```python
from build123d import *

# Parameters (mm, degrees)
F0_R     = 44
F1_DEPTH = 2
F0_R_2   = 1.5
F2_DEPTH = 1


# Not quite as in the source:
# - a fillet or chamfer that OpenCascade refuses, or shapes differently, is made with other operations: its cross-section is extruded or revolved along the edge and cut away or added


with BuildPart() as f1:
    # F0 (on Front) → F1 (new body)
    with BuildSketch(Plane.XZ):
        with BuildLine():
            Line((-77.5, -50), (77.5, -50))
            Line((77.5, -50), (77.5, -40))
            Line((77.5, -40), (72.5, -40))
            ThreePointArc((72.5, -40), (67.5, -35), (72.5, -30))
            Line((72.5, -30), (77.5, -30))
            Line((77.5, -30), (77.5, 30))
            Line((77.5, 30), (72.5, 30))
            ThreePointArc((72.5, 30), (67.5, 35), (72.5, 40))
            Line((72.5, 40), (77.5, 40))
            Line((77.5, 40), (77.5, 50))
            Line((77.5, 50), (-77.5, 50))
            Line((-77.5, 50), (-77.5, 40))
            Line((-77.5, 40), (-72.5, 40))
            ThreePointArc((-72.5, 40), (-67.5, 35), (-72.5, 30))
            Line((-72.5, 30), (-77.5, 30))
            Line((-77.5, 30), (-77.5, -30))
            Line((-77.5, -30), (-72.5, -30))
            ThreePointArc((-72.5, -30), (-67.5, -35), (-72.5, -40))
            Line((-72.5, -40), (-77.5, -40))
            Line((-77.5, -40), (-77.5, -50))
        make_face()
        with BuildLine():
            Line((43.5, -46), (-43.5, -46))
            ThreePointArc((-43.5, -46), (-47.767766953, -47.767766953), (-46, -43.5))
            Line((-46, -43.5), (-46, 43.5))
            ThreePointArc((-46, 43.5), (-47.767766953, 47.767766953), (-43.5, 46))
            Line((-43.5, 46), (43.5, 46))
            ThreePointArc((43.5, 46), (46, 48.5), (48.5, 46))
            ThreePointArc((48.5, 46), (47.767766953, 44.232233047), (46, 43.5))
            Line((46, 43.5), (46, -43.5))
            ThreePointArc((46, -43.5), (47.767766953, -44.232233047), (48.5, -46))
            ThreePointArc((48.5, -46), (46, -48.5), (43.5, -46))
        make_face(mode=Mode.SUBTRACT)
        with BuildLine():
            ThreePointArc((-46, -43.5), (-44.232233047, -44.232233047), (-43.5, -46))
            Line((-43.5, -46), (43.5, -46))
            ThreePointArc((43.5, -46), (44.232233047, -44.232233047), (46, -43.5))
            Line((46, -43.5), (46, 43.5))
            ThreePointArc((46, 43.5), (44.232233047, 44.232233047), (43.5, 46))
            Line((43.5, 46), (-43.5, 46))
            ThreePointArc((-43.5, 46), (-44.232233047, 44.232233047), (-46, 43.5))
            Line((-46, 43.5), (-46, -43.5))
        make_face()
        Circle(F0_R, mode=Mode.SUBTRACT)
    extrude(amount=F1_DEPTH)

    # F0 (on Front) → F2 (join)
    with BuildSketch(Plane.XZ):
        with BuildLine():
            Line((-77.5, -30), (-77.5, -40))
            Line((-77.5, -40), (-72.5, -40))
            ThreePointArc((-72.5, -40), (-67.5, -35), (-72.5, -30))
            Line((-72.5, -30), (-77.5, -30))
        make_face()
        with Locations((-72.5, -35)):
            Circle(F0_R_2, mode=Mode.SUBTRACT)
        with BuildLine():
            Line((-77.5, 40), (-77.5, 30))
            Line((-77.5, 30), (-72.5, 30))
            ThreePointArc((-72.5, 30), (-67.5, 35), (-72.5, 40))
            Line((-72.5, 40), (-77.5, 40))
        make_face()
        with Locations((-72.5, 35)):
            Circle(F0_R_2, mode=Mode.SUBTRACT)
        with BuildLine():
            Line((72.5, 30), (77.5, 30))
            Line((77.5, 30), (77.5, 40))
            Line((77.5, 40), (72.5, 40))
            ThreePointArc((72.5, 40), (67.5, 35), (72.5, 30))
        make_face()
        with Locations((72.5, 35)):
            Circle(F0_R_2, mode=Mode.SUBTRACT)
        with BuildLine():
            Line((72.5, -40), (77.5, -40))
            Line((77.5, -40), (77.5, -30))
            Line((77.5, -30), (72.5, -30))
            ThreePointArc((72.5, -30), (67.5, -35), (72.5, -40))
        make_face()
        with Locations((72.5, -35)):
            Circle(F0_R_2, mode=Mode.SUBTRACT)
        with BuildLine():
            ThreePointArc((-43.5, 46), (-47.767766953, 47.767766953), (-46, 43.5))
            Line((-46, 43.5), (-46, 44.5))
            ThreePointArc((-46, 44.5), (-47.0606601718, 47.0606601718), (-44.5, 46))
            Line((-44.5, 46), (-43.5, 46))
        make_face()
        with BuildLine():
            Line((-46, 44.5), (-46, 43.5))
            ThreePointArc((-46, 43.5), (-44.232233047, 44.232233047), (-43.5, 46))
            Line((-43.5, 46), (-44.5, 46))
            ThreePointArc((-44.5, 46), (-44.9393398282, 44.9393398282), (-46, 44.5))
        make_face()
        with BuildLine():
            Line((46, 44.5), (46, 43.5))
            ThreePointArc((46, 43.5), (47.767766953, 44.232233047), (48.5, 46))
            ThreePointArc((48.5, 46), (46, 48.5), (43.5, 46))
            Line((43.5, 46), (44.5, 46))
            ThreePointArc((44.5, 46), (46, 47.5), (47.5, 46))
            ThreePointArc((47.5, 46), (47.0606601718, 44.9393398282), (46, 44.5))
        make_face()
        with BuildLine():
            ThreePointArc((43.5, 46), (44.232233047, 44.232233047), (46, 43.5))
            Line((46, 43.5), (46, 44.5))
            ThreePointArc((46, 44.5), (44.9393398282, 44.9393398282), (44.5, 46))
            Line((44.5, 46), (43.5, 46))
        make_face()
        with BuildLine():
            Line((44.5, -46), (43.5, -46))
            ThreePointArc((43.5, -46), (46, -48.5), (48.5, -46))
            ThreePointArc((48.5, -46), (47.767766953, -44.232233047), (46, -43.5))
            Line((46, -43.5), (46, -44.5))
            ThreePointArc((46, -44.5), (47.0606601718, -44.9393398282), (47.5, -46))
            ThreePointArc((47.5, -46), (46, -47.5), (44.5, -46))
        make_face()
        with BuildLine():
            ThreePointArc((46, -43.5), (44.232233047, -44.232233047), (43.5, -46))
            Line((43.5, -46), (44.5, -46))
            ThreePointArc((44.5, -46), (44.9393398282, -44.9393398282), (46, -44.5))
            Line((46, -44.5), (46, -43.5))
        make_face()
        with BuildLine():
            Line((-44.5, -46), (-43.5, -46))
            ThreePointArc((-43.5, -46), (-44.232233047, -44.232233047), (-46, -43.5))
            Line((-46, -43.5), (-46, -44.5))
            ThreePointArc((-46, -44.5), (-44.9393398282, -44.9393398282), (-44.5, -46))
        make_face()
        with BuildLine():
            ThreePointArc((-46, -43.5), (-47.767766953, -47.767766953), (-43.5, -46))
            Line((-43.5, -46), (-44.5, -46))
            ThreePointArc((-44.5, -46), (-47.0606601718, -47.0606601718), (-46, -44.5))
            Line((-46, -44.5), (-46, -43.5))
        make_face()
    extrude(amount=F2_DEPTH)

    # F3: fillet of radius 5 on 1 edges, made by hand

    # F3_s1 → F3_t2 (revolve, cut)
    with BuildSketch(Plane.XY):
        with BuildLine():
            ThreePointArc((48, -2), (45.7639320225, -1.472135955), (44, 0))
            Line((44, 0), (44, -2))
            Line((44, -2), (48, -2))
        make_face()
    revolve(axis=Axis((0, -2, 0), (0, -1, 0)), mode=Mode.SUBTRACT)


solid = f1.part
```
Work out the finished part from the listing and answer in its coordinate system (mm). A direction names the side the tool comes from. Coordinates: 2 decimals unless noted, no trailing zeros. Loops run counter-clockwise (first coordinate to the right, second up) from the corner with the lowest first, then second, coordinate; pieces in that order, holes last. Notation, with made-up numbers: (-19, 44) - (24, 44) arc R23 ccw to (24, 53) - close; hole circle Ø5 at (21, 28.5). An arc over 180 degrees is marked (long way). Use a Markdown table: item, result.
Item 1: Consider probe 1 along X at (y, z) = (-0.25, 46); probe 2 along X at (y, z) = (-1.25, 46); probe 3 along Z at (x, y) = (-46, -0.5). Determine where each line is inside the solid, lowest interval first. Write a range as from..to.
Evaluation:
| item | result |
|---|---|
| probe 1 | x = -77.5..-47.5, -44.5..44.5, 47.5..77.5 |
| probe 2 | x = -77.5..-48.5, -43.5..43.5, 48.5..77.5 |
| probe 3 | z = -50..-47.5, -44.5..44.5, 47.5..50 |
Item 2: Find section A-A, the plane y = -1.45. Determine the outline of the cut face in (x, z).
Evaluation:
| item | result |
|---|---|
| outline | (-77.5, -50) - (77.5, -50) - (77.5, -40) - (72.5, -40) arc R5 cw to (72.5, -30) - (77.5, -30) - (77.5, 30) - (72.5, 30) arc R5 cw to (72.5, 40) - (77.5, 40) - (77.5, 50) - (-77.5, 50) - (-77.5, 40) - (-72.5, 40) arc R5 cw to (-72.5, 30) - (-77.5, 30) - (-77.5, -30) - (-72.5, -30) arc R5 cw to (-72.5, -40) - (-77.5, -40) - close; hole circle Ø5 at (-46, -46); hole circle Ø5 at (-46, 46); hole circle Ø91.44 at (0, 0); hole circle Ø5 at (46, -46); hole circle Ø5 at (46, 46) |
Item 3: Given pin 1 Ø1.5 at (x, z) = (-45, 46.5) entering from -Y; pin 2 Ø2.5 at (x, z) = (72.5, 35) entering from +Y, each flat-ended and moving along its own axis, determine where each tip first touches the part or whether it passes through.
Evaluation:
| item | result |
|---|---|
| pin 1 | stops at y = -1 |
| pin 2 | passes through |
Item 4: The mould has two halves that part along Z. Classify faces 1 (the flat face through (-1, 0, 45)), 2 (the cylindrical face through (67.5, -1.5, 34.9)): +Z half, -Z half, draft (parallel to the pull), parting line (faces both ways), or undercut.
Evaluation:
| item | result |
|---|---|
| face 1 | draft |
| face 2 | undercut |
Item 5: For faces 3 (the flat face through (-18, -2, 45)), 4 (the flat face through (74, -1, 36)), 5 (the cylindrical face through (-71.114, -0.493, 34.425)), 6 (the flat face through (-44, -1, -46)), 7 (the flat face through (-74, -1, -36)), determine the directions among +Z, -Z, +X, -X, +Y, -Y from which every point of the face is accessible in a straight line to the end or side of a thin tool.
Evaluation:
| item | result |
|---|---|
| face 3 | +Z, -Z, +X, -X, -Y |
| face 4 | +X, -Y |
| face 5 | +Y, -Y |
| face 6 | -Y |
| face 7 | -X, -Y |
